from build123d import *

# Parameters (mm, degrees)
F0_R     = 4
F1_DEPTH = 203.2
F2_R     = 6.35
F3_DEPTH = 1.27
F4_R     = 4
F5_DEPTH = 12.7


with BuildPart() as f1:
    # F0 (on Right) → F1 (new body)
    with BuildSketch(Plane.YZ):
        Circle(F0_R)
    extrude(amount=F1_DEPTH)

    # F2 (on Right) → F3 (join)
    with BuildSketch(Plane.YZ):
        Circle(F2_R)
    extrude(amount=F3_DEPTH)

    # F4 (on Right) → F5 (join)
    with BuildSketch(Plane.YZ):
        Circle(F4_R)
    extrude(amount=-F5_DEPTH)


solid = f1.part
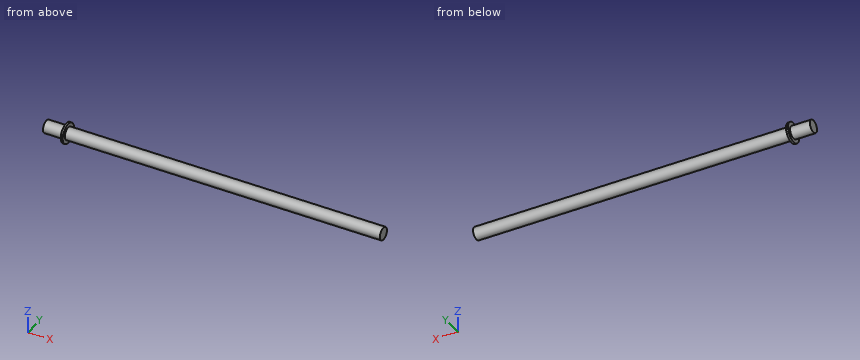
Source: CAD feature listing. Evaluate the final solid. Frame: model axes, mm. Give positions to 0.01 mm unless a question says otherwise; leave off trailing zeros. Order: outer loops, then holes, each group sorted by start corner. A loop starts at its lowest first (then second) coordinate and runs counter-clockwise, first axis right, second up. Notation, with made-up numbers: (50.25, -1.5) -> (102.25, -1.5) arc R15 cw to (102.25, 23.5) -> close; hole circle Ø9 at (77.5, 29). An arc over 180 degrees is marked (long way). Write item = value, one per line.
Q1. Cut plane C-C, the plane x = 183. Output: boundary loops of the cut face in (y, z).
Data:
outline = circle Ø8 at (0, 0)
Q2. Pin query (flat end, axial travel): pin 1 (1 mm diameter, centred on x = 93.5, z = 1.5, fed in from -Y); pin 2 (1 mm diameter, centred on y = -4, z = -3.5, fed in from +X). Return the tip coordinate at first contact, or that it passes through.
Data:
pin_1 = -3.87
pin_2 = 1.27
Q3. Cut plane A-A, the plane y = 0. Output: boundary loops of the cut face in (x, z).
Data:
outline = (-12.7, -4) -> (0, -4) -> (0, -6.35) -> (1.27, -6.35) -> (1.27, -4) -> (203.2, -4) -> (203.2, 4) -> (1.27, 4) -> (1.27, 6.35) -> (0, 6.35) -> (0, 4) -> (-12.7, 4) -> close
Q4. Material intervals for line 1 (X direction, y = -3, z = 3); line 2 (Y direction, x = 185, z = -0.5), sorted ascending. Write a range as from..to.
Data:
line_1 = 0..1.27
line_2 = -3.97..3.97
